Design review of the part built by this model. Coordinates are the model's own, in mm. A direction names the side the tool comes from. Give positions to 0.01 mm unless a question says otherwise; leave off trailing zeros. Write each loop counter-clockwise with the first axis right and the second up, starting at its lowest first coordinate (ties: lowest second). Pieces come first, ordered by that corner, then holes. Notation, with made-up numbers: M -18.75,79 L 13.25,79 A27 ccw 13.25,104 Z; hole C 81,-31.75 d6. An arc over 180 degrees is marked long. Answer in a Markdown table with one row per item.
```python
from build123d import *

# Parameters (mm, degrees)
F0_R     = 11.673828125
F1_DEPTH = 60
F3_START = -3.8
F2_W     = 52
F2_H     = 28.3295102417
F3_DEPTH = 9.3
F4_R     = 11.673828125
F5_DEPTH = 1


with BuildPart() as f1:
    # F0 (on Right) → F1 (new body)
    with BuildSketch(Plane.YZ):
        Circle(F0_R)
        with BuildLine():
            ThreePointArc((-5.4563251713, -9.173828125), (-5.2768707474, 9.2782132955), (10.673828125, 0))
            ThreePointArc((10.673828125, 0), (9.2782132955, -5.2768707474), (5.4563251713, -9.173828125))
            ThreePointArc((5.4563251713, -9.173828125), (0, -10.673828125), (-5.4563251713, -9.173828125))
        make_face(mode=Mode.SUBTRACT)
        with BuildLine():
            Line((5.4563251713, -9.173828125), (-5.4563251713, -9.173828125))
            ThreePointArc((-5.4563251713, -9.173828125), (0, -10.673828125), (5.4563251713, -9.173828125))
        make_face()
    extrude(amount=F1_DEPTH)

    # F2 (on Top) → F3 (cut)
    with BuildSketch(Plane.XY.offset(F3_START)):
        with Locations((30, 0)):
            Rectangle(F2_W, F2_H)
    extrude(amount=-F3_DEPTH, mode=Mode.SUBTRACT)

    # F4 (on face) → F5 (join)
    with BuildSketch(Plane.YZ):
        Circle(F4_R)
    extrude(amount=F5_DEPTH)


solid = f1.part
```
1) Add section B-B (z = -4.75). Write out the cut boundary in (x, y).
Geometry says:
| item | result |
|---|---|
| outline | M 0,-10.66 L 4,-10.66 L 4,-9.56 L 1,-9.56 L 1,9.56 L 4,9.56 L 4,10.66 L 0,10.66 Z; M 56,-10.66 L 60,-10.66 L 60,-9.56 L 56,-9.56 Z; M 56,9.56 L 60,9.56 L 60,10.66 L 56,10.66 Z |
2) Insertion check: P1, Ø13, axis at y = 0, z = 0, coming from the +X side; P2, Ø3, axis at x = 38, y = -5, coming from the -Z side; P3, Ø0.9, axis at x = 32, y = 10, coming from the -Z side. Each pin has a flat end and moves straight along its axis. Give the tip position at first contact, or say it passes through.
Geometry says:
| item | result |
|---|---|
| P1 | x = 1 |
| P2 | z = 8.47 |
| P3 | z = -3.8 |
3) For faces 4 (the face through (29.6, -10.5, -3.8)), 5 (the face through (1, 0, 1)), 6 (the face through (29.58, -1.52, 11.574)), list the 3-axis set-ups (+Z, -Z, +X, -X, +Y, -Y) from which the entire face can be reached by the end or side of a thin tool; tool diameter is ignored.
Geometry says:
| item | result |
|---|---|
| face 4 | -Z, +Y, -Y |
| face 5 | +X |
| face 6 | +X, -X |
4) To check wall thickness, follow probe 1 along X at (y, z) = (-4.5, -9.5); probe 2 along X at (y, z) = (4.25, -6.5); probe 3 along Y at (x, z) = (37.5, -0.75). State the ranges of each line that lie inside material, in increasing order. Write a range as [from, to].
Geometry says:
| item | result |
|---|---|
| probe 1 | [0, 4], [56, 60] |
| probe 2 | [0, 1] |
| probe 3 | [-11.65, -10.65], [10.65, 11.65] |
5) The part is to be moulded in two halves that separate along X. For faces 1 (the face through (29.6, 10.5, -3.8)), 2 (the face through (0, 0, 0)), 3 (the face through (58, 0, -9.174)), say which applies: released by +X, released by -X, zero draft, split by the parting line, or undercut.
Geometry says:
| item | result |
|---|---|
| face 1 | undercut |
| face 2 | released by -X |
| face 3 | zero draft |
6) Add section C-C (x = 36.5). Write out the cut boundary in (y, z).
Geometry says:
| item | result |
|---|---|
| outline | M -11.04,-3.8 L -9.97,-3.8 A10.67 cw long 9.97,-3.8 L 11.04,-3.8 A11.67 ccw long Z |
7) Add section A-A (y = 0). Write out the cut boundary in (x, z).
Geometry says:
| item | result |
|---|---|
| outline | M 0,-11.67 L 4,-11.67 L 4,-9.17 L 1,-9.17 L 1,10.67 L 60,10.67 L 60,11.67 L 0,11.67 Z; M 56,-11.67 L 60,-11.67 L 60,-9.17 L 56,-9.17 Z |
8) Add section D-D (z = 2.75). Write out the cut boundary in (x, y), and give its area (3 significant figures).
Geometry says:
| item | result |
|---|---|
| outline | M 0,-11.35 L 60,-11.35 L 60,-10.31 L 1,-10.31 L 1,10.31 L 60,10.31 L 60,11.35 L 0,11.35 Z |
| area | 144 mm^2 |
